```python
from build123d import *

# Parameters (mm, degrees)
SKETCH1_W           = 120
SKETCH1_H           = 100
BOSS_EXTRUDE1_DEPTH = 20
SKETCH6_W           = 110
SKETCH6_H           = 40
CUT_EXTRUDE1_DEPTH  = 20
SKETCH6_3_W         = 5
SKETCH6_3_H         = 40
BOSS_EXTRUDE4_DEPTH = 20
SKETCH14_W          = 5
SKETCH14_H          = 5
CUT_EXTRUDE2_DEPTH  = 10
SKETCH15_W          = 10
SKETCH15_H          = 10
CUT_EXTRUDE3_DEPTH  = 10


with BuildPart() as part:
    # Sketch1 → Boss-Extrude1 (new body)
    with BuildSketch(Plane(origin=(0, 0, 0), x_dir=(1, 0, 0), z_dir=(0, 1, 0))):
        Rectangle(SKETCH1_W, SKETCH1_H)
    extrude(amount=BOSS_EXTRUDE1_DEPTH)

    # Sketch6 → Cut-Extrude1 (cut)
    with BuildSketch(Plane.XZ):
        with Locations((0, 25)):
            Rectangle(SKETCH6_W, SKETCH6_H)
    extrude(amount=-CUT_EXTRUDE1_DEPTH, mode=Mode.SUBTRACT)

    # Sketch6_3 → Boss-Extrude4 (add)
    with BuildSketch(Plane.XZ):
        with Locations((-52.5, 25)):
            Rectangle(SKETCH6_3_W, SKETCH6_3_H)
        with Locations((52.5, 25)):
            Rectangle(SKETCH6_3_W, SKETCH6_3_H)
    extrude(amount=-BOSS_EXTRUDE4_DEPTH)

    # Sketch14 → Cut-Extrude2 (cut)
    with BuildSketch(Plane(origin=(0, 20, 0), x_dir=(1, 0, 0), z_dir=(0, 1, 0))):
        with Locations((-57.5, -7.820888862)):
            Rectangle(SKETCH14_W, SKETCH14_H)
        Polygon((-50, -0.320888862), (-60, -0.320888862), (-60, -5.320888862), (-55, -5.320888862), (-55, -10.320888862), (-50, -10.320888862), (-50, -5), align=None)
        Polygon((60, -5.320888862), (60, -0.320888862), (50, -0.320888862), (50, -5), (50, -10.320888862), (55, -10.320888862), (55, -5.320888862), align=None)
        with Locations((57.5, -7.820888862)):
            Rectangle(SKETCH14_W, SKETCH14_H)
    extrude(amount=-CUT_EXTRUDE2_DEPTH, mode=Mode.SUBTRACT)

    # Sketch15 → Cut-Extrude3 (cut)
    with BuildSketch(Plane(origin=(0, 20, 0), x_dir=(1, 0, 0), z_dir=(0, 1, 0))):
        with Locations((-55, 45)):
            Rectangle(SKETCH15_W, SKETCH15_H)
        with Locations((55, 45)):
            Rectangle(SKETCH15_W, SKETCH15_H)
        with Locations((55, -45)):
            Rectangle(SKETCH15_W, SKETCH15_H)
        with Locations((-55, -45)):
            Rectangle(SKETCH15_W, SKETCH15_H)
    extrude(amount=-CUT_EXTRUDE3_DEPTH, mode=Mode.SUBTRACT)


solid = part.part
```
Here's how the part is built. I have some questions about the finished solid (model axes, mm). A direction names the side the tool comes from. Round coordinates to 2 decimals unless told otherwise and drop trailing zeros. Write each loop counter-clockwise with the first axis right and the second up, starting at its lowest first coordinate (ties: lowest second). Pieces come first, ordered by that corner, then holes. Notation, with made-up numbers: M 59,-12 L 99,-12 A28 cw 99,10 Z; hole C -3.75,-2.5 d3. An arc over 180 degrees is marked long. Answer as CSV lines item,"result". Start each with the question number.
1. Suppose I cut it at D-D on z = -42. Write out the boundary of the cut face in (x, y).
2. Suppose I cut it at B-B on x = -47.5. Write out the boundary of the cut face in (y, z), then the cut area to 3 significant figures.
3. On a 3-axis mill with a long thin cutter (end or side, diameter ignored), from which of +Z, -Z, +X, -X, +Y, -Y can I reach the whole of each face in a straight line? I mean faces 1 (the flat face through (55, 15, 10.321)), 2 (the flat face through (55, 15, 40)), 3 (the flat face through (-55, 10, -45)), 4 (the flat face through (-50, 15, 48)), 5 (the flat face through (55, 15, 0.321)). Say none if no direction works.
4. Suppose I cut it at A-A on y = 14.25. Write out the boundary of the cut face in (x, z), then the cut area to 3 significant figures.
5. I need wall thicknesses on probe 1 along Z at (x, y) = (38, 15); probe 2 along X at (y, z) = (1.25, 37). Which ranges of each line are inside material? Lowest first, please.
6. Suppose I cut it at C-C on y = 2.5. Write out the boundary of the cut face in (x, z).
7. I'm going to push flat-ended pins straight in: pin 1 Ø5 at (x, z) = (-53, 4) entering from +Y; pin 2 Ø3 at (x, y) = (-57, 14) entering from -Z; pin 3 Ø2.5 at (y, z) = (14, 2) entering from +X. Where does each tip first touch, or does it pass through?
8. Thinking about a two-plate mould opening in Z: for faces 6 (the flat face through (55, 10, 5)), 7 (the flat face through (-55, 15, 40)), 8 (the flat face through (55, 20, 25)), which applies, released by +Z, released by -Z, zero draft, split by the parting line, or undercut?
Check result:
1,outline,"M -60,0 L 60,0 L 60,10 L 50,10 L 50,20 L -50,20 L -50,10 L -60,10 Z"
2,outline,"M 0,-50 L 20,-50 L 20,5 L 0,5 Z; M 0,45 L 20,45 L 20,50 L 0,50 Z"
2,area,"1,200 mm2"
3,face 1,"+X, -X, +Y"
3,face 2,"+Z, +X, -X, +Y"
3,face 3,"-Z, -X, +Y"
3,face 4,"+Z, -X, +Y"
3,face 5,"+X, +Y"
4,outline,"M -60,-40 L -50,-40 L -50,-50 L 50,-50 L 50,-40 L 60,-40 L 60,0.32 L 50,0.32 L 50,5 L -50,5 L -50,0.32 L -60,0.32 Z; M -60,10.32 L -50,10.32 L -50,40 L -60,40 Z; M -50,45 L 50,45 L 50,50 L -50,50 Z; M 50,10.32 L 60,10.32 L 60,40 L 50,40 Z"
4,area,"7,400 mm2"
5,probe 1,"z = -50 to 5, 45 to 50"
5,probe 2,"x = -60 to -50, 50 to 60"
6,outline,"M -60,-50 L 60,-50 L 60,50 L -60,50 Z; hole M -50,5 L 50,5 L 50,45 L -50,45 Z"
7,pin 1,"stops at y = 10"
7,pin 2,"stops at z = -40"
7,pin 3,"stops at x = 50"
8,face 6,"undercut"
8,face 7,"released by +Z"
8,face 8,"zero draft"
